Could you check a few things on this model? Use its own coordinates, in mm. Face numbers are marked on the shaded views. A direction names the side the tool comes from. Give positions to 0.01 mm unless a question says otherwise; leave off trailing zeros. Loops run counter-clockwise (first coordinate to the right, second up) from the corner with the lowest first, then second, coordinate; pieces in that order, holes last. Notation, with made-up numbers: (-32.75, 84) - (-26.75, 84) arc R18 ccw to (-26.75, 90) - close; hole circle Ø4 at (16.5, -24.75). An arc over 180 degrees is marked (long way). Use CSV: the item, a comma, the result in double quotes.
from build123d import *

# Parameters (mm, degrees)
F1_DEPTH = 93.6625
F3_DEPTH = 0.508


with BuildPart() as f1:
    # F0 (on Right) → F1 (new body)
    with BuildSketch(Plane.YZ):
        Polygon((1.27, -9.525), (1.27, 1.5875), (-1.27, 1.5875), (-1.27, 9.525), (-2.54, 9.525), (-2.54, -9.525), align=None)
    extrude(amount=F1_DEPTH)

    # F2 (on face) → F3 (join)
    with BuildSketch(Plane.XZ.offset(2.54)):
        with BuildLine():
            Line((93.6625, 9.525), (93.6625, 7.62))
            ThreePointArc((93.6625, 7.62), (95.0095384182, 8.1779615818), (95.5675, 9.525))
            ThreePointArc((95.5675, 9.525), (93.6625, 11.43), (91.7575, 9.525))
            Line((91.7575, 9.525), (93.6625, 9.525))
        make_face()
        with BuildLine():
            ThreePointArc((91.7575, -9.525), (93.6625, -11.43), (95.5675, -9.525))
            ThreePointArc((95.5675, -9.525), (95.0095384182, -8.1779615818), (93.6625, -7.62))
            Line((93.6625, -7.62), (93.6625, -9.525))
            Line((93.6625, -9.525), (91.7575, -9.525))
        make_face()
        with BuildLine():
            ThreePointArc((0, -7.62), (-1.3470384182, -10.8720384182), (1.905, -9.525))
            Line((1.905, -9.525), (0, -9.525))
            Line((0, -9.525), (0, -7.62))
        make_face()
        with BuildLine():
            Line((0, 9.525), (1.905, 9.525))
            ThreePointArc((1.905, 9.525), (-1.3470384182, 10.8720384182), (0, 7.62))
            Line((0, 7.62), (0, 9.525))
        make_face()
    extrude(amount=-F3_DEPTH)


solid = f1.part
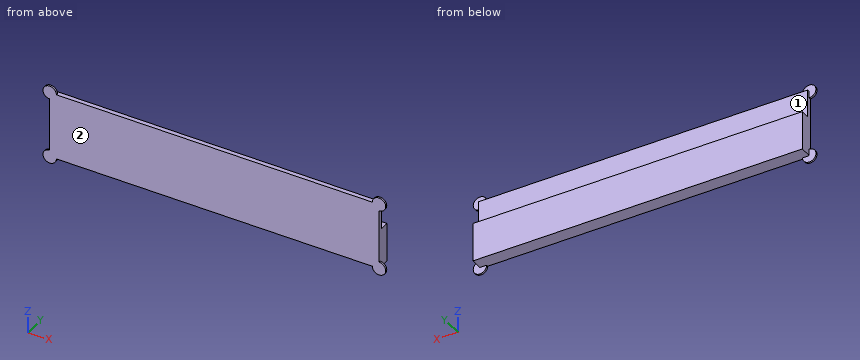
1) Suppose I cut it at B-B (x = 54.5). Please give me the cut outline in (y, z) (1 decimal).
Answer below:
outline,"(-2.5, -9.5) - (1.3, -9.5) - (1.3, 1.6) - (-1.3, 1.6) - (-1.3, 9.5) - (-2.5, 9.5) - close"
2) Suppose I cut it at A-A (z = -0.25). Please give me the cut outline in (x, y).
Answer below:
outline,"(0, -2.54) - (93.66, -2.54) - (93.66, 1.27) - (0, 1.27) - close"
3) Suppose I cut it at C-C (y = 0). Please give me the cut outline in (x, z) (1 decimal), plus the area to 3 significant figures.
Answer below:
outline,"(0, -9.5) - (93.7, -9.5) - (93.7, 1.6) - (0, 1.6) - close"
area,"1,040 mm2"
4) I need wall thicknesses on line 1 along Z through (x, y) = (36.5, 1.05) (1 decimal); line 2 along Z through (x, y) = (31, -1.45) (3 decimals); line 3 along X through (y, z) = (-1.15, -0.75). Which ranges of each line are inside material? Lowest first, please.
Answer below:
line 1,"z = -9.5 to 1.6"
line 2,"z = -9.525 to 9.525"
line 3,"x = 0 to 93.66"
5) Which directions (+Z, -Z, +X, -X, +Y, -Y) give clear straight access to the entire face, cutting with the end or side of a thin tool? Please do the marked faces 1 and 2.
Answer below:
face 1,"+Z, +X, -X, +Y"
face 2,"+Z, -Z, +X, -X, -Y"
6) I'm going to push flat-ended pins straight in: P1, Ø6.5, axis at x = 24.5, z = 6.5, coming from the +Y side; P2, Ø1, axis at x = 59, y = -2, coming from the +Z side (3 decimals); P3, Ø2, axis at y = 0, z = 7.5, coming from the +X side; P4, Ø1.1, axis at y = -0.5, z = -2.5, coming from the -X side. Where does each tip first touch, or does it pass through?
Answer below:
P1,"stops at y = -1.27"
P2,"stops at z = 9.525"
P3,"passes through"
P4,"stops at x = 0"
